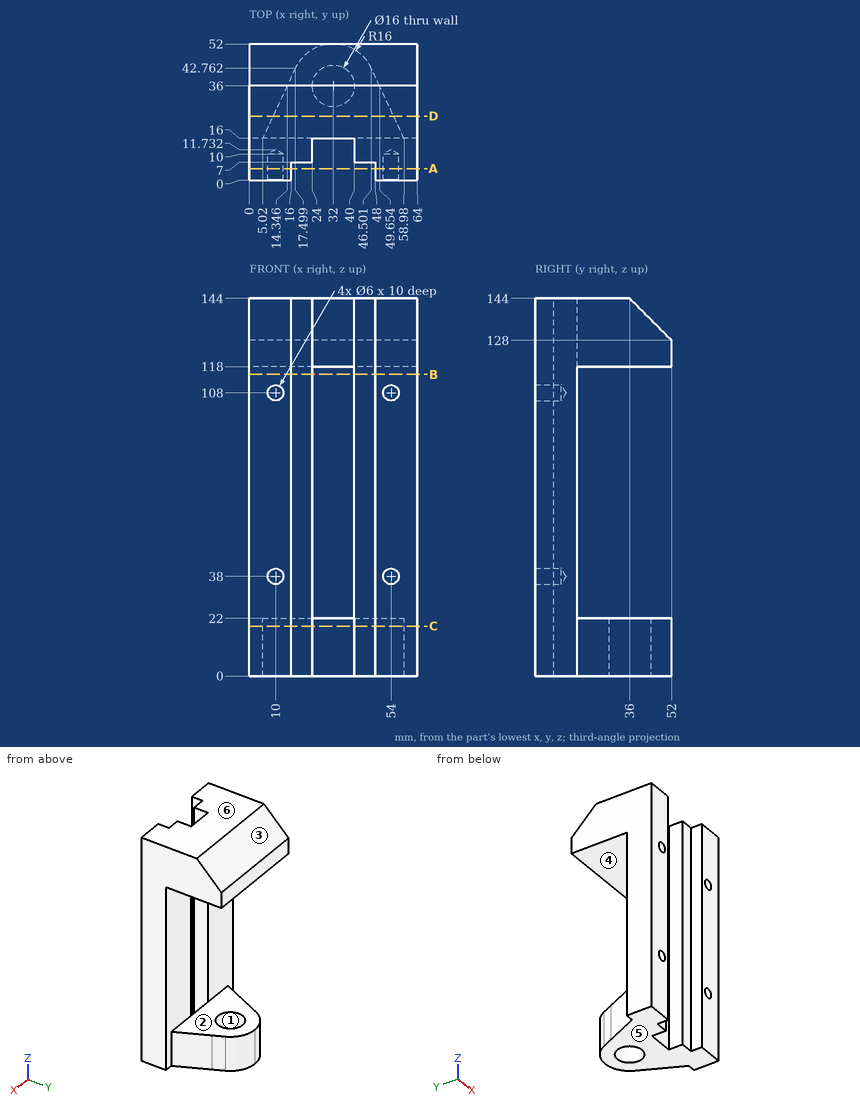
Job drawing, mm, ordinate dimensions from the low corner. One solid piece. A direction names the side the tool comes from. Give positions to 0.01 mm unless a question says otherwise; leave off trailing zeros. Write each loop counter-clockwise with the first axis right and the second up, starting at its lowest first coordinate (ties: lowest second). Pieces come first, ordered by that corner, then holes. Notation, with made-up numbers: M 34,64 L 51,64 A26 ccw 51,84 Z; hole C 19,70 d9. An arc over 180 degrees is marked long. One line per item, written item: value. Start each with the question number.
Q1. Two-plate mould, pull along Z, no slides. Class the marked faces 4, 5 and 6: +Z half, -Z half, draft (parallel to the pull), parting line (faces both ways), or undercut.
Q2. Saw through at A-A, the plane y = 4.5. Write the cut outline in (x, z).
Q3. Saw through at C-C, the plane z = 19. Write the cut outline in (x, y).
Q4. Saw through at B-B, the plane z = 115. Write the cut outline in (x, y).
Q5. Probe probe 1 along Z at (x, y) = (54, 7.25); probe 2 along X at (y, z) = (4, 108); probe 3 along Z at (x, y) = (47.5, 27). List the from-to ranges inside material, lowest first. Write a range as [from, to].
Q6. 3-axis set-ups, long thin cutter, end or side, ignore diameter. For the marked faces 1, 2 and 3: which of +Z, -Z, +X, -X, +Y, -Y reach the whole face in a straight line?
Q7. Saw through at D-D, the plane y = 24.5. Write the cut outline in (x, z).
Q8. Drop flat-ended pins along their axis: pin 1 Ø7 at (x, z) = (49, 43) entering from +Y; pin 2 Ø17.5 at (x, z) = (33, 126.5) entering from -Y. Give the stop position or say it passes through.
Output values:
1. face 4: undercut
1. face 5: -Z half
1. face 6: +Z half
2. outline: M 0,0 L 16,0 L 16,144 L 0,144 Z; M 48,0 L 64,0 L 64,144 L 48,144 Z; hole C 10,38 d6; hole C 10,108 d6; hole C 54,38 d6; hole C 54,108 d6
3. outline: M 0,0 L 16,0 L 16,7 L 24,7 L 24,16 L 40,16 L 40,7 L 48,7 L 48,0 L 64,0 L 64,16 L 58.98,16 L 46.5,42.76 A16 ccw 17.5,42.76 L 5.02,16 L 0,16 Z; hole C 32,36 d16
4. outline: M 0,0 L 16,0 L 16,7 L 24,7 L 24,16 L 0,16 Z; M 40,7 L 48,7 L 48,0 L 64,0 L 64,16 L 40,16 Z
5. probe 1: z = [0, 35], [41, 105], [111, 144]
5. probe 2: x = [0, 7], [13, 16], [48, 51], [57, 64]
5. probe 3: z = [0, 22], [118, 144]
6. face 1: -Z
6. face 2: +X, -X, +Y
6. face 3: +Z, +X, -X, +Y
7. outline: M 0,118 L 64,118 L 64,144 L 0,144 Z; M 8.98,0 L 55.02,0 L 55.02,22 L 8.98,22 Z
8. pin 1: stops at y = 16
8. pin 2: stops at y = 7
